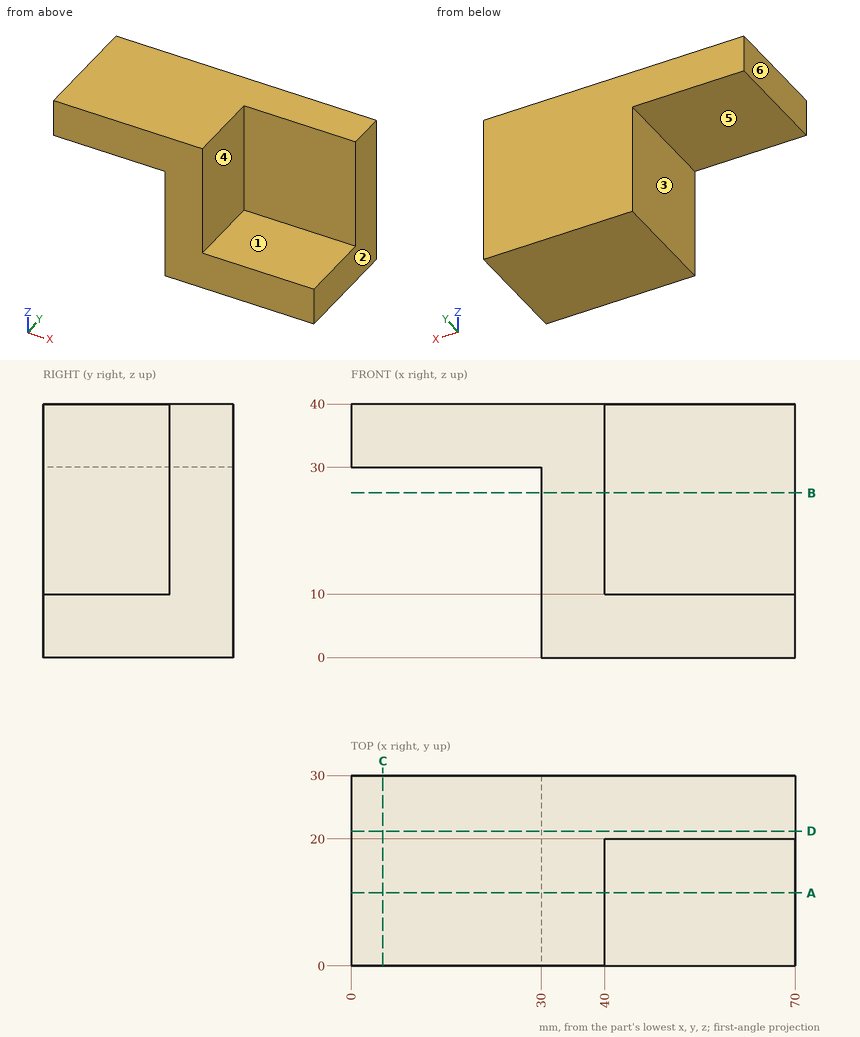
Here's the drawing with two shaded views (mm, measured from the low corner). I have some questions. A direction names the side the tool comes from. Coordinates: 2 decimals unless noted, no trailing zeros. Order: outer loops, then holes, each group sorted by start corner. A loop starts at its lowest first (then second) coordinate and runs counter-clockwise, first axis right, second up.
Item 1: Thinking about a two-plate mould opening in X: for the marked faces 1, 2 and 3, which applies, pulls with the +X half, pulls with the -X half, needs draft (parallel to the pull), parting line crosses it, or undercut?
Response values:
face 1: needs draft
face 2: pulls with the +X half
face 3: pulls with the -X half
Item 2: I'm going to push flat-ended pins straight in: pin 1 Ø10 at (x, y) = (61.5, 12.5) entering from +Z; pin 2 Ø15 at (x, y) = (16, 18) entering from -Z; pin 3 Ø1.5 at (y, z) = (18, 34) entering from +X. Where does each tip first touch, or does it pass through?
Response values:
pin 1: stops at z = 10
pin 2: stops at z = 30
pin 3: stops at x = 40
Item 3: I need wall thicknesses on probe 1 along X at (y, z) = (23.5, 15.5); probe 2 along Y at (x, z) = (44, 31.5); probe 3 along Z at (x, y) = (64.5, 4.75). Which ranges of each line are inside material? Lowest first, please.
Response values:
probe 1: x = 30 to 70
probe 2: y = 20 to 30
probe 3: z = 0 to 10
Item 4: If we section it at B-B, the plane z = 26: List the corners of the cut face in (x, y) for me.
Response values:
outline: (30, 0) - (40, 0) - (40, 20) - (70, 20) - (70, 30) - (30, 30) - close
Item 5: If we section it at A-A, the plane y = 11.5: List the corners of the cut face in (x, z) for me.
Response values:
outline: (0, 30) - (30, 30) - (30, 0) - (70, 0) - (70, 10) - (40, 10) - (40, 40) - (0, 40) - close
Item 6: If we section it at D-D, the plane y = 21.25: List the corners of the cut face in (x, z) for me.
Response values:
outline: (0, 30) - (30, 30) - (30, 0) - (70, 0) - (70, 40) - (0, 40) - close
Item 7: If we section it at C-C, the plane x = 5: List the corners of the cut face in (y, z) for me, then the cut area to 3 significant figures.
Response values:
outline: (0, 30) - (30, 30) - (30, 40) - (0, 40) - close
area: 300 mm2
Item 8: Which directions (+Z, -Z, +X, -X, +Y, -Y) give clear straight access to the entire face, cutting with the end or side of a thin tool? Please do the marked faces 4, 5 and 6.
Response values:
face 4: +Z, +X, -Y
face 5: -Z, -X, +Y, -Y
face 6: +Z, -Z, -X, +Y, -Y
